Geometry: final body of the model. Coordinates: model frame, mm. Face numbers are marked on the shaded views. A direction names the side the tool comes from. Round coordinates to 2 decimals unless told otherwise and drop trailing zeros. Loops run counter-clockwise (first coordinate to the right, second up) from the corner with the lowest first, then second, coordinate; pieces in that order, holes last. Notation, with made-up numbers: (3.25, 70.25) - (47.25, 70.25) arc R10 ccw to (47.25, 77.25) - close; hole circle Ø11 at (85.25, 14.25). An arc over 180 degrees is marked (long way). Write item = value, one per line. Start each with the question number.
Item 1: Section A-A (z = 4). Return loops of the section in (x, y).
Item 2: Section C-C (z = -2.25). Return loops of the section in (x, y).
Item 3: Draft query along Y for the marked faces 1, 2 and 3. Return one class per face: pulls with the +Y half, pulls with the -Y half, needs draft (parallel to the pull), parting line crosses it, or undercut.
Item 4: First-contact query: pin 1 (12 mm diameter, centred on x = -10, y = 2.5, fed in from +Z) (3 decimals); pin 2 (2.5 mm diameter, centred on x = 1, y = 7.5, fed in from -Z); pin 3 (4 mm diameter, centred on y = -10.5, z = -1, fed in from -X); pin 4 (1 mm diameter, centred on x = 4, z = -6.5, fed in from -Y). Flat tips, straight axial feed; report the tip coordinate or a pass-through.
Item 5: Access query for the marked faces 4 and 5. Directions: +Z, -Z, +X, -X, +Y, -Y. A direction counts if a zero-diameter tool reaches every point of the face in a straight line with its end or side. Return the directions, or none.
Item 6: Line query: line 1 (Y direction, x = 2, z = 2.25); line 2 (Y direction, x = 2.5, z = 3.25); line 3 (Z direction, x = -6, y = 8). Output: solid intervals per line, ascending. Write a range as from..to.
from build123d import *

# Parameters (mm, degrees)
F0_R          = 4.7625
F1_DEPTH      = 9.525
F1_DEPTH_BACK = 6.35
F3_DEPTH      = 9.526
F4_R          = 15.24
F5_DEPTH      = 15.24
F6_R          = 2.413
F7_DEPTH      = 13.97
F8_SIZE2      = 9.525
F8_SIZE       = 5.08
F9_R          = 5.08


with BuildPart() as f1:
    # F0 (on Top) → F1 (new body, two sides)
    with BuildSketch(Plane.XY) as f1_sk:
        Circle(F0_R)
    extrude(amount=F1_DEPTH)
    extrude(f1_sk.sketch, amount=-F1_DEPTH_BACK)

    # F2 (on Top) → F3 (cut, through all)
    with BuildSketch(Plane.XY):
        with BuildLine():
            ThreePointArc((1.9843134833, -2.25), (2.7343134833, -1.2343134833), (3, 0))
            ThreePointArc((3, 0), (2.7343134833, 1.2343134833), (1.9843134833, 2.25))
            Line((1.9843134833, 2.25), (-1.9843134833, 2.25))
            ThreePointArc((-1.9843134833, 2.25), (-3, 0), (-1.9843134833, -2.25))
            Line((-1.9843134833, -2.25), (1.9843134833, -2.25))
        make_face()
    extrude(amount=F3_DEPTH, mode=Mode.SUBTRACT)

    # F4 (on Top) → F5 (join)
    with BuildSketch(Plane.XY):
        Circle(F4_R)
    extrude(amount=-F5_DEPTH)

    # F6 (on face) → F7 (cut)
    with BuildSketch(Plane(origin=(0, 0, -15.24), x_dir=(1, 0, 0), z_dir=(0, 0, -1))):
        with Locations((1.0674559099, -7.8653953575)):
            Circle(F6_R)
        with Locations((6.2779042355, 4.8571416142)):
            Circle(F6_R)
        with Locations((-7.3453601454, 3.0082537434)):
            Circle(F6_R)
    extrude(amount=-F7_DEPTH, mode=Mode.SUBTRACT)

    # F8
    f8_edges = [f1.edges().sort_by_distance(p)[0] for p in [
        (-15.24, 0, 0),
    ]]
    f8_side = f1.faces().sort_by_distance((-14.808948, 0, 0))[0]
    chamfer(f8_edges, length=F8_SIZE, length2=F8_SIZE2, reference=f8_side)

    # F9
    f9_edges = [f1.edges().sort_by_distance(p)[0] for p in [
        (-4.7625, 0, 0),
    ]]
    fillet(f9_edges, radius=F9_R)


solid = f1.part
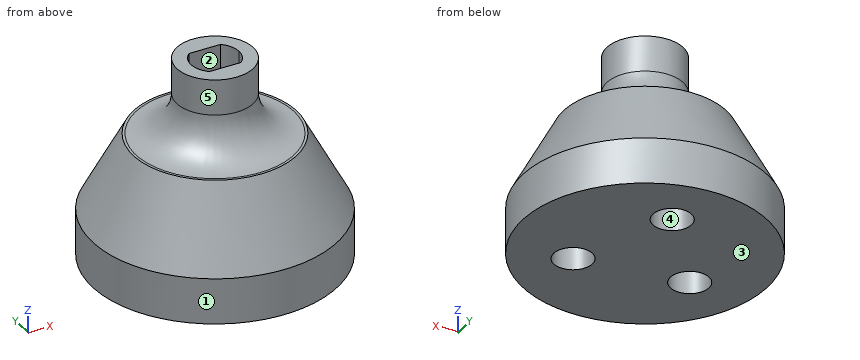
Taken from the geometry:
q1.outline = circle Ø9.76 at (0, 0); hole (-1.98, -2.25) - (1.98, -2.25) arc R3 ccw to (1.98, 2.25) - (-1.98, 2.25) arc R3 ccw to start
q2.outline = circle Ø22.72 at (0, 0); hole circle Ø4.83 at (-7.35, -3.01); hole circle Ø4.83 at (1.07, 7.87); hole circle Ø4.83 at (6.28, -4.86)
q3.face_1 = parting line crosses it
q3.face_2 = undercut
q3.face_3 = needs draft
q4.pin_1 = 9.525
q4.pin_2 = -1.27
q4.pin_3 = -7.02
q4.pin_4 = -13.34
q5.face_4 = -Z
q5.face_5 = +Z
q6.line_1 = -5.26..-2.24, 2.24..5.26
q6.line_2 = -4.45..-1.66, 1.66..4.45
q6.line_3 = -15.24..0
